from build123d import *

# Parameters (mm, degrees)
SKETCH1_W           = 19
SKETCH1_H           = 19
SKETCH1_W_2         = 15
SKETCH1_H_2         = 15
BOSS_EXTRUDE1_DEPTH = 149
SKETCH2_R           = 2
CUT_EXTRUDE1_DEPTH  = 10
SKETCH5_R           = 2
CUT_EXTRUDE2_DEPTH  = 151.506644372
SKETCH6_R           = 2
CUT_EXTRUDE3_DEPTH  = 151.506644372


with BuildPart() as part:
    # Sketch1 → Boss-Extrude1 (new body)
    with BuildSketch(Plane.XY):
        Rectangle(SKETCH1_W, SKETCH1_H)
        Rectangle(SKETCH1_W_2, SKETCH1_H_2, mode=Mode.SUBTRACT)
    extrude(amount=BOSS_EXTRUDE1_DEPTH)

    # Sketch2 → Cut-Extrude1 (cut)
    with BuildSketch(Plane(origin=(9.5, 0, 0), x_dir=(0, 0, -1), z_dir=(1, 0, 0))):
        with Locations((-138.5, 4.5)):
            Circle(SKETCH2_R)
        with Locations((-138.5, -4.5)):
            Circle(SKETCH2_R)
    extrude(amount=-CUT_EXTRUDE1_DEPTH, mode=Mode.SUBTRACT)

    # Sketch5 → Cut-Extrude2 (cut, through all)
    with BuildSketch(Plane(origin=(0, 9.5, 0), x_dir=(1, 0, 0), z_dir=(0, 1, 0))):
        with Locations(Location((0.61, -89.67, 0), (0, 0, 270))):
            Circle(SKETCH5_R)
    extrude(amount=-CUT_EXTRUDE2_DEPTH, mode=Mode.SUBTRACT)

    # Sketch6 → Cut-Extrude3 (cut, through all)
    with BuildSketch(Plane.ZY.offset(9.5)):
        with Locations((93.91, 2)):
            Circle(SKETCH6_R)
        with Locations((123.91, 2)):
            Circle(SKETCH6_R)
    extrude(amount=-CUT_EXTRUDE3_DEPTH, mode=Mode.SUBTRACT)


solid = part.part
Input: part model. Units: mm. Frame: model coordinates. A direction names the side the tool comes from. Coordinates: 2 decimals unless noted, no trailing zeros. Loops run counter-clockwise (first coordinate to the right, second up) from the corner with the lowest first, then second, coordinate; pieces in that order, holes last.
Q1. Cut plane B-B (x = -3.75). Output: boundary loops of the cut face in (y, z).
Q2. Contact query for flat-ended pins moving along their axis: pin 1 (6.5 mm diameter, centred on x = 0.61, z = 89.67, fed in from +Y); pin 2 (2.5 mm diameter, centred on y = 2, z = 123.91, fed in from +X). Output: stop coordinate, or through.
Q3. Set-up query: faces 4 (the face through (8.514, 4.588, 140.498)), 5 (the face through (8.486, 2.601, 95.818)), 6 (the face through (7.5, 0, 73)). Return all of +Z, -Z, +X, -X, +Y, -Y with unobstructed straight access to the full face (end or side cutting, diameter ignored); none if empty.
Q4. Draft query along Y for faces 1 (the face through (8.514, -4.412, 140.498)), 2 (the face through (0, -9.5, 73)), 3 (the face through (9.5, 0, 73)). Return one class per face: +Y half, -Y half, draft (parallel to the pull), parting line (faces both ways), or undercut.
Q5. Material intervals for line 1 (X direction, y = 2.5, z = 133.5); line 2 (Y direction, x = 8.2, z = 93.91), sorted ascending.
Q6. Cut plane A-A (z = 93.91). Output: boundary loops of the cut face in (x, y), then the cut area to 3 significant figures.
Working result:
1. outline: (-9.5, 0) - (-7.5, 0) - (-7.5, 149) - (-9.5, 149) - close; (7.5, 0) - (9.5, 0) - (9.5, 149) - (7.5, 149) - close
2. pin 1: stops at y = 9.5
2. pin 2: passes through
3. face 4: +X
3. face 5: +X, -X
3. face 6: +Z, -Z
4. face 1: undercut
4. face 2: -Y half
4. face 3: draft
5. line 1: x = -9.5 to -7.5, 7.5 to 9.5
5. line 2: y = -9.5 to 0, 4 to 9.5
6. outline: (-9.5, -9.5) - (9.5, -9.5) - (9.5, 0) - (7.5, 0) - (7.5, -7.5) - (-7.5, -7.5) - (-7.5, 0) - (-9.5, 0) - close; (-9.5, 4) - (-7.5, 4) - (-7.5, 7.5) - (7.5, 7.5) - (7.5, 4) - (9.5, 4) - (9.5, 9.5) - (-9.5, 9.5) - close
6. area: 120 mm2
